from build123d import *

# Parameters (mm, degrees)
SKETCH1_W                                         = 69.85
SKETCH1_H                                         = 127
BOSS_EXTRUDE1_DEPTH                               = 3.175
SKETCH2_R                                         = 2.5
BOSS_EXTRUDE2_DEPTH                               = 3.175
M3X0_5_TAPPED_HOLE1_D                             = 2.5
SKETCH5_R                                         = 1.5
BOSS_EXTRUDE3_DEPTH                               = 3.175
CSK_FOR_4_FLAT_HEAD_MACHINE_SCREW_100_D           = 3.4544
CSK_FOR_4_FLAT_HEAD_MACHINE_SCREW_100_CSINK_D     = 5.715
CSK_FOR_4_FLAT_HEAD_MACHINE_SCREW_100_CSINK_ANGLE = 100
FILLET1_R                                         = 5.08


with BuildPart() as part:
    # Sketch1 → Boss-Extrude1 (new body)
    with BuildSketch(Plane(origin=(0, 0, 0), x_dir=(1, 0, 0), z_dir=(0, 1, 0))):
        with Locations((34.925, 63.5)):
            Rectangle(SKETCH1_W, SKETCH1_H)
    extrude(amount=BOSS_EXTRUDE1_DEPTH)

    # Sketch2 → Boss-Extrude2 (add)
    with BuildSketch(Plane(origin=(0, 3.175, 0), x_dir=(1, 0, 0), z_dir=(0, 1, 0))):
        with Locations(Location((10.795, 100.33, 0), (0, 0, 90))):
            Circle(SKETCH2_R)
        with Locations(Location((59.055, 99.06, 0), (0, 0, 90))):
            Circle(SKETCH2_R)
        with Locations(Location((15.875, 46.19857895, 0), (0, 0, 90))):
            Circle(SKETCH2_R)
        with Locations(Location((43.815, 46.19857895, 0), (0, 0, 90))):
            Circle(SKETCH2_R)
        with Locations(Location((10.795, 20.102862456, 0), (0, 0, 90))):
            Circle(SKETCH2_R)
        with Locations(Location((59.055, 27.216985797, 0), (0, 0, 90))):
            Circle(SKETCH2_R)
    extrude(amount=BOSS_EXTRUDE2_DEPTH)

    # M3x0.5 Tapped Hole1 (through all)
    with Locations(Plane(origin=(0, 6.35, 0), x_dir=(1, 0, 0), z_dir=(0, 1, 0))):
        with Locations((10.795, 100.33), (15.875, 46.19857895), (43.815, 46.19857895), (10.795, 20.102862456)):
            Hole(M3X0_5_TAPPED_HOLE1_D / 2)

    # Sketch5 → Boss-Extrude3 (add)
    with BuildSketch(Plane(origin=(0, 6.35, 0), x_dir=(1, 0, 0), z_dir=(0, 1, 0))):
        with Locations(Location((59.055, 99.06, 0), (0, 0, 270))):
            Circle(SKETCH5_R)
        with Locations(Location((59.055, 27.216985797, 0), (0, 0, 270))):
            Circle(SKETCH5_R)
    extrude(amount=BOSS_EXTRUDE3_DEPTH)

    # CSK for #4 Flat Head Machine Screw (100)1 (through all)
    with Locations(Plane(origin=(0, 3.175, 0), x_dir=(1, 0, 0), z_dir=(0, 1, 0))):
        with Locations((3.175, 123.825), (66.675, 123.825), (66.675, 3.175), (3.175, 3.175)):
            CounterSinkHole(CSK_FOR_4_FLAT_HEAD_MACHINE_SCREW_100_D / 2, CSK_FOR_4_FLAT_HEAD_MACHINE_SCREW_100_CSINK_D / 2, counter_sink_angle=CSK_FOR_4_FLAT_HEAD_MACHINE_SCREW_100_CSINK_ANGLE)

    # Fillet1
    # the kernel refuses this fillet: 5.08 mm, written as the material it adds along each edge
    with BuildSketch(Plane(origin=(10.795, 3.175, -100.33), x_dir=(0, 0, -1), z_dir=(1, 0, 0))) as fillet1_piece_1:
        with BuildLine():
            CenterArc((7.209286039, 5.08), FILLET1_R, 202.024312837, 67.975687163)
            Line((2.5, 3.175), (2.405814279, 3.1369))
            ThreePointArc((2.405814279, 3.1369), (2.3984, 1.5875), (2.3984, 0))
            Line((2.3984, 0), (2.5, -0.1016))
            Line((2.5, -0.1016), (7.209286039, -0.1016))
            Line((7.209286039, -0.1016), (7.209286039, 0))
        make_face()
    revolve(axis=Axis((10.795, 3.175, -100.33), (0, 1, 0)))
    with BuildSketch(Plane(origin=(59.055, 3.175, -99.06), x_dir=(0, 0, -1), z_dir=(1, 0, 0))) as fillet1_piece_2:
        with BuildLine():
            CenterArc((7.209286039, 5.08), FILLET1_R, 202.024312837, 67.975687163)
            Line((2.5, 3.175), (2.405814279, 3.1369))
            ThreePointArc((2.405814279, 3.1369), (2.3984, 1.5875), (2.3984, 0))
            Line((2.3984, 0), (2.5, -0.1016))
            Line((2.5, -0.1016), (7.209286039, -0.1016))
            Line((7.209286039, -0.1016), (7.209286039, 0))
        make_face()
    revolve(axis=Axis((59.055, 3.175, -99.06), (0, 1, 0)))
    with BuildSketch(Plane(origin=(15.875, 3.175, -46.19857895), x_dir=(0, 0, -1), z_dir=(1, 0, 0))) as fillet1_piece_3:
        with BuildLine():
            CenterArc((7.209286039, 5.08), FILLET1_R, 202.024312837, 67.975687163)
            Line((2.5, 3.175), (2.405814279, 3.1369))
            ThreePointArc((2.405814279, 3.1369), (2.3984, 1.5875), (2.3984, 0))
            Line((2.3984, 0), (2.5, -0.1016))
            Line((2.5, -0.1016), (7.209286039, -0.1016))
            Line((7.209286039, -0.1016), (7.209286039, 0))
        make_face()
    revolve(axis=Axis((15.875, 3.175, -46.19857895), (0, 1, 0)))
    with BuildSketch(Plane(origin=(43.815, 3.175, -46.19857895), x_dir=(0, 0, -1), z_dir=(1, 0, 0))) as fillet1_piece_4:
        with BuildLine():
            CenterArc((7.209286039, 5.08), FILLET1_R, 202.024312837, 67.975687163)
            Line((2.5, 3.175), (2.405814279, 3.1369))
            ThreePointArc((2.405814279, 3.1369), (2.3984, 1.5875), (2.3984, 0))
            Line((2.3984, 0), (2.5, -0.1016))
            Line((2.5, -0.1016), (7.209286039, -0.1016))
            Line((7.209286039, -0.1016), (7.209286039, 0))
        make_face()
    revolve(axis=Axis((43.815, 3.175, -46.19857895), (0, 1, 0)))
    with BuildSketch(Plane(origin=(10.795, 3.175, -20.102862456), x_dir=(0, 0, -1), z_dir=(1, 0, 0))) as fillet1_piece_5:
        with BuildLine():
            CenterArc((7.209286039, 5.08), FILLET1_R, 202.024312837, 67.975687163)
            Line((2.5, 3.175), (2.405814279, 3.1369))
            ThreePointArc((2.405814279, 3.1369), (2.3984, 1.5875), (2.3984, 0))
            Line((2.3984, 0), (2.5, -0.1016))
            Line((2.5, -0.1016), (7.209286039, -0.1016))
            Line((7.209286039, -0.1016), (7.209286039, 0))
        make_face()
    revolve(axis=Axis((10.795, 3.175, -20.102862456), (0, 1, 0)))
    with BuildSketch(Plane(origin=(59.055, 3.175, -27.216985797), x_dir=(0, 0, -1), z_dir=(1, 0, 0))) as fillet1_piece_6:
        with BuildLine():
            CenterArc((7.209286039, 5.08), FILLET1_R, 202.024312837, 67.975687163)
            Line((2.5, 3.175), (2.405814279, 3.1369))
            ThreePointArc((2.405814279, 3.1369), (2.3984, 1.5875), (2.3984, 0))
            Line((2.3984, 0), (2.5, -0.1016))
            Line((2.5, -0.1016), (7.209286039, -0.1016))
            Line((7.209286039, -0.1016), (7.209286039, 0))
        make_face()
    revolve(axis=Axis((59.055, 3.175, -27.216985797), (0, 1, 0)))


solid = part.part
Part model, mm, in its own coordinate system. A direction names the side the tool comes from. Coordinates: 2 decimals unless noted, no trailing zeros. Loops run counter-clockwise (first coordinate to the right, second up) from the corner with the lowest first, then second, coordinate; pieces in that order, holes last. Notation, with made-up numbers: M 18.25,86.25 L 33.25,86.25 A28 cw 33.25,118.25 Z; hole C 61.25,-10 d10. An arc over 180 degrees is marked long. Use a Markdown table: item, result. Add a question column.
Q1. Probe L1, parallel to Z at x = 10, y = 0.5; L2, parallel to Z at x = 13, y = 4; L3, parallel to Y at x = 15.5, z = -71 (3 decimals). List the from-to ranges inside material, lowest first.
Q2. Mould opens along Z. For faces 4 (the flat face through (43, 6.35, -45)), 5 (the cylindrical face through (58.14, 7.92, -100.25)), 6 (the flat face through (34, 2, 0)) say: +Z half, -Z half, draft (parallel to the pull), parting line (faces both ways), or undercut.
Q3. Which spindle directions (+Z, -Z, +X, -X, +Y, -Y) get a long thin tool onto all of the face, cutting with end or side? Do faces 1 (the flat face through (10, 6.35, -99)), 2 (the flat face through (59, 9.525, -99)), 3 (the cylindrical face through (57.59, 7.92, -27.54)). Say none if no direction does.
Q4. Pin check, flat tips, straight feed: P1, Ø2, axis at x = 66.675, z = -3.175, coming from the -Y side; P2, Ø4, axis at x = 42.5, z = -47, coming from the +Y side; P3, Ø1.5, axis at x = 12, z = -101, coming from the +Y side; P4, Ø12, axis at x = 48, z = -69, coming from the +Y side (3 decimals). Stop position of each tip, or through.
Q5. Cut at C-C (x = 26.5). Write the cut outline in (y, z) (3 decimals).
Q6. Cut at B-B (z = -68.5). Write the cut outline in (x, y) (3 decimals), and give its area (3 significant figures).
Q7. Cut at A-A (y = 4.5). Give the number of separate pieces and of enclosed holes in the cut face, and give its area (3 significant figures).
Worked out:
| question | item | result |
|---|---|---|
| 1 | L1 | z = -127 to -101.29, -99.37 to -21.07, -19.14 to 0 |
| 1 | L2 | z = -104.18 to -96.48, -49.57 to -42.82, -23.95 to -16.26 |
| 1 | L3 | y = 0 to 3.175 |
| 2 | face 4 | draft |
| 2 | face 5 | undercut |
| 2 | face 6 | +Z half |
| 3 | face 1 | +Z, -Z, -X, +Y |
| 3 | face 2 | +Z, -Z, +X, -X, +Y |
| 3 | face 3 | +Y |
| 4 | P1 | passes through |
| 4 | P2 | stops at y = 6.35 |
| 4 | P3 | stops at y = 6.35 |
| 4 | P4 | stops at y = 3.175 |
| 5 | outline | M 0,-127 L 3.175,-127 L 3.175,0 L 0,0 Z |
| 6 | outline | M 0,0 L 69.85,0 L 69.85,3.175 L 0,3.175 Z |
| 6 | area | 222 mm2 |
| 7 | separate pieces | 6 |
| 7 | enclosed holes | 4 |
| 7 | area | 251 mm2 |
